Can you work these out from the model? Positions are in its coordinate system, mm. A direction names the side the tool comes from. Give positions to 0.01 mm unless a question says otherwise; leave off trailing zeros. Loops run counter-clockwise (first coordinate to the right, second up) from the corner with the lowest first, then second, coordinate; pieces in that order, holes last. Notation, with made-up numbers: (15, 87) - (34, 87) arc R22 ccw to (34, 109) - close; hole circle Ø10 at (-32.5, -12). An arc over 180 degrees is marked (long way). Write item = value, one per line.
from build123d import *

# Parameters (mm, degrees)
ESQUISSE1_W             = 25
ESQUISSE1_H             = 16
BOSS_EXTRU_1_DEPTH      = 9
ESQUISSE2_R             = 3.5
ENL_V_MAT_EXTRU_1_DEPTH = 32.016124839
BOSS_EXTRU_2_DEPTH      = 4
BOSS_EXTRU_2_DEPTH_BACK = 29
ESQUISSE5_W             = 7.685000099
ESQUISSE5_H             = 9
ESQUISSE3_W             = 30
ESQUISSE3_H             = 3.5
ENL_V_MAT_EXTRU_3_DEPTH = 35.322004603


with BuildPart() as part:
    # Esquisse1 → Boss.-Extru.1 (new body)
    with BuildSketch(Plane(origin=(0, 0, 0), x_dir=(1, 0, 0), z_dir=(0, 1, 0))):
        with Locations((12.5, 8)):
            Rectangle(ESQUISSE1_W, ESQUISSE1_H)
    extrude(amount=BOSS_EXTRU_1_DEPTH)

    # Esquisse2 → Enlèv. mat.-Extru.1 (cut, through all)
    with BuildSketch(Plane(origin=(25, 0, 0), x_dir=(0, 0, -1), z_dir=(1, 0, 0))):
        with Locations((4.5, 4.5)):
            Circle(ESQUISSE2_R)
    extrude(amount=-ENL_V_MAT_EXTRU_1_DEPTH, mode=Mode.SUBTRACT)

    # Esquisse5 → Boss.-Extru.2 (add, two sides: drawn at the far end of the back side and taken through both)
    with BuildSketch(Plane(origin=(25, 0, 0), x_dir=(0, 0, -1), z_dir=(1, 0, 0)).offset(-BOSS_EXTRU_2_DEPTH_BACK)):
        with Locations((12.157499951, 4.5)):
            Rectangle(ESQUISSE5_W, ESQUISSE5_H)
    extrude(amount=BOSS_EXTRU_2_DEPTH + BOSS_EXTRU_2_DEPTH_BACK)

    # Esquisse3 → Enlèv. mat.-Extru.3 (cut, through all)
    with BuildSketch(Plane(origin=(0, 9, 0), x_dir=(1, 0, 0), z_dir=(0, 1, 0))):
        with Locations((12.5, 11.640847207)):
            Rectangle(ESQUISSE3_W, ESQUISSE3_H)
    extrude(amount=-ENL_V_MAT_EXTRU_3_DEPTH, mode=Mode.SUBTRACT)


solid = part.part
Q1. Imagine slicing it at C-C, the plane z = -4.5. Write out the boundary of the cut face in (x, y).
Output:
outline = (0, 0) - (25, 0) - (25, 1) - (0, 1) - close; (0, 8) - (25, 8) - (25, 9) - (0, 9) - close
Q2. Which directions (+Z, -Z, +X, -X, +Y, -Y) give clear straight access to the entire face, cutting with the end or side of a thin tool? Please do faces 4 (the flat face through (12, 4, -16)), 5 (the flat face through (25, 6, -1)), 6 (the flat face through (-2, 4, -8.315)), 7 (the flat face through (12, 5, -13.391)).
Output:
face_4 = -Z, +X, -X, +Y, -Y
face_5 = +Z, +X, +Y, -Y
face_6 = +Z, -X, +Y, -Y
face_7 = +Y, -Y
Q3. For pin 1 (4 mm diameter, centred on y = 4.5, z = -4.5, fed in from -X); pin 2 (2 mm diameter, centred on x = -2.5, y = 4, fed in from +Z) (3 decimals); pin 3 (1.5 mm diameter, centred on y = 4.5, z = -8, fed in from -X), each with a flat end and sliding along its axis, tell me the tip position at first contact or that it passes through.
Output:
pin_1 = through
pin_2 = -8.315
pin_3 = -4
Q4. Imagine slicing it at A-A, the plane x = 18.5. Write out the boundary of the cut face in (y, z), then the cut area to 3 significant figures.
Output:
outline = (0, -16) - (9, -16) - (9, -13.39) - (0, -13.39) - close; (0, -9.89) - (9, -9.89) - (9, 0) - (0, 0) - close; hole circle Ø7 at (4.5, -4.5)
area = 74.0 mm2
Q5. Imagine slicing it at B-B, the plane y = 5.25. Write out the boundary of the cut face in (x, z) (3 decimals), then the cut area to 3 significant figures.
Output:
outline = (-4, -16) - (29, -16) - (29, -8.315) - (25, -8.315) - (25, -7.919) - (0, -7.919) - (0, -8.315) - (-4, -8.315) - close; (0, -1.081) - (25, -1.081) - (25, 0) - (0, 0) - close; hole (-2.5, -13.391) - (27.5, -13.391) - (27.5, -9.891) - (-2.5, -9.891) - close
area = 186 mm2
Q6. I need wall thicknesses on L1, parallel to X at y = 3.5, z = -10.25; L2, parallel to Y at x = 11.5, z = -4.5; L3, parallel to Z at x = 27, y = 5 (3 decimals). Which ranges of each line are inside material? Lowest first, please.
Output:
L1 = -4 to -2.5, 27.5 to 29
L2 = 0 to 1, 8 to 9
L3 = -16 to -13.391, -9.891 to -8.315
Q7. We'd pull the mould along X, two halves only. Please class faces 1 (the flat face through (12, 0, -8)), 2 (the flat face through (12, 5, -9.891)), 3 (the flat face through (0, 6, -1)): released by +X, released by -X, zero draft, split by the parting line, or undercut.
Output:
face_1 = zero draft
face_2 = undercut
face_3 = released by -X
Q8. Imagine slicing it at D-D, the plane y = 2.75. Write out the boundary of the cut face in (x, z) (3 decimals).
Output:
outline = (-4, -16) - (29, -16) - (29, -8.315) - (25, -8.315) - (25, -7.531) - (0, -7.531) - (0, -8.315) - (-4, -8.315) - close; (0, -1.469) - (25, -1.469) - (25, 0) - (0, 0) - close; hole (-2.5, -13.391) - (27.5, -13.391) - (27.5, -9.891) - (-2.5, -9.891) - close
